Geometry: final body of the model. Coordinates: model frame, mm. A direction names the side the tool comes from. Give positions to 0.01 mm unless a question says otherwise; leave off trailing zeros. Loops run counter-clockwise (first coordinate to the right, second up) from the corner with the lowest first, then second, coordinate; pieces in that order, holes last. Notation, with made-up numbers: (7.5, 59.25) - (42.5, 59.25) arc R17 ccw to (42.5, 83.25) - close; hole circle Ø3 at (51, -39). An arc over 180 degrees is marked (long way). Use CSV: the item, a comma, the result in double quotes. Start each with the question number.
```python
from build123d import *

# Parameters (mm, degrees)
F0_W          = 136.4381015301
F0_H          = 72.4301114678
F1_DEPTH      = 25.4
F2_R          = 23.2656169201
F3_DEPTH      = 36.322
F5_DEPTH      = 25.4
F5_DEPTH_BACK = 25.4


with BuildPart() as f1:
    # F0 (on Top) → F1 (new body)
    with BuildSketch(Plane.XY):
        Rectangle(F0_W, F0_H)
    extrude(amount=F1_DEPTH)

    # F2 (on face) → F3 (join)
    with BuildSketch(Plane.XY.offset(25.4)):
        Circle(F2_R)
    extrude(amount=F3_DEPTH)

    # F4 (on Front) → F5 (cut, two sides)
    with BuildSketch(Plane.XZ) as f5_sk:
        Polygon((54.1822127998, 69.6227326989), (-68.4997886419, 65.6924173236), (54.1822127998, 42.1105287969), align=None)
    extrude(amount=-F5_DEPTH, mode=Mode.SUBTRACT)
    extrude(f5_sk.sketch, amount=F5_DEPTH_BACK, mode=Mode.SUBTRACT)


solid = f1.part
```
Item 1: Section D-D (x = 36). Output: boundary loops of the cut face in (y, z), plus the area to 3 significant figures.
Item 2: Ray query, probe 1 along Z at (x, y) = (-47, -5.5); probe 2 along X at (y, z) = (0, 31); probe 3 along Y at (x, z) = (12, 42). Return the intervals inside material, ascending.
Item 3: Section C-C (z = 43). Output: boundary loops of the cut face in (x, y).
Item 4: Pin query (flat end, axial travel): pin 1 Ø8 at (y, z) = (18, 42.5) entering from +X; pin 2 Ø5 at (y, z) = (14.5, 46.5) entering from -X; pin 3 Ø2 at (x, y) = (-52, 3.5) entering from -Z; pin 4 Ø10 at (x, y) = (-54.5, 1.5) entering from +Z. Return the tip coordinate at first contact, or that it passes through.
Item 5: Reachability of faces 1 (the cylindrical face through (-23.243, 1.023, 37.467)), 2 (the flat face through (-1, -36.215, 13)) from +Z, -Z, +X, -X, +Y, -Y: full face, straight path, thin tool, end or side. Return the list, or none.
Item 6: Section A-A (y = 0). Output: boundary loops of the cut face in (x, z), plus the area to 3 significant figures.
Item 7: Section B-B (x = -11). Output: boundary loops of the cut face in (y, z), plus the area to 3 significant figures.
Outcome:
1,outline,"(-36.22, 0) - (36.22, 0) - (36.22, 25.4) - (-36.22, 25.4) - close"
1,area,"1,840 mm2"
2,probe 1,"z = 0 to 25.4"
2,probe 2,"x = -23.27 to 23.27"
2,probe 3,"y = -19.93 to 19.93"
3,outline,"circle Ø46.53 at (0, 0)"
4,pin 1,"stops at x = 18.58"
4,pin 2,"stops at x = -19.93"
4,pin 3,"stops at z = 0"
4,pin 4,"stops at z = 25.4"
5,face 1,"+Z"
5,face 2,"+Z, -Z, +X, -X, -Y"
6,outline,"(-68.22, 0) - (68.22, 0) - (68.22, 25.4) - (23.27, 25.4) - (23.27, 48.05) - (-23.27, 57) - (-23.27, 25.4) - (-68.22, 25.4) - close"
6,area,"4,730 mm2"
7,outline,"(-36.22, 0) - (36.22, 0) - (36.22, 25.4) - (20.5, 25.4) - (20.5, 54.64) - (-20.5, 54.64) - (-20.5, 25.4) - (-36.22, 25.4) - close"
7,area,"3,040 mm2"
